Answer from the drawing. Dimensions are ordinates in mm from the lowest x, y and z of the part. A direction names the side the tool comes from. Round coordinates to 2 decimals unless told otherwise and drop trailing zeros. Order: outer loops, then holes, each group sorted by start corner. A loop starts at its lowest first (then second) coordinate and runs counter-clockwise, first axis right, second up. Notation, with made-up numbers: (50, -29) -> (54, -29) arc R15 ccw to (54, 0) -> close; hole circle Ø3 at (-3, 35.5). An arc over 180 degrees is marked (long way). Use a Markdown table: item, result. Add a question column.
1. Section D-D, the plane x = 12 is taken. Give the vertices of the cut face in (y, z), then the cut area to 3 significant figures.
2. The mould has two halves that part along Z. Classify the marked faces 3, 4 and 5: +Z half, -Z half, draft (parallel to the pull), parting line (faces both ways), or undercut.
3. Consider L1, parallel to Z at x = 52, y = 18.5; L2, parallel to X at y = 31, z = 96; L3, parallel to X at y = 28, z = 99. Determine where each line is inside the solid, lowest interval first. Write a range as [from, to].
4. Section C-C, the plane z = 93 is taken. Give the vertices of the cut face in (x, y).
5. For the marked faces 1 and 2, determine the directions among +Z, -Z, +X, -X, +Y, -Y from which every point of the face is accessible in a straight line to the end or side of a thin tool.
6. Given pin 1 (3 mm diameter, centred on x = 7.5, y = 39, fed in from +Z); pin 2 (5 mm diameter, centred on x = 24, z = 34.5, fed in from +Y); pin 3 (10 mm diameter, centred on x = 30.5, z = 37, fed in from +Y), each flat-ended and moving along its own axis, determine where each tip first touches the part or whether it passes through.
7. Section A-A, the plane y = 32 is taken. Give the vertices of the cut face in (x, z), then the cut area to 3 significant figures.
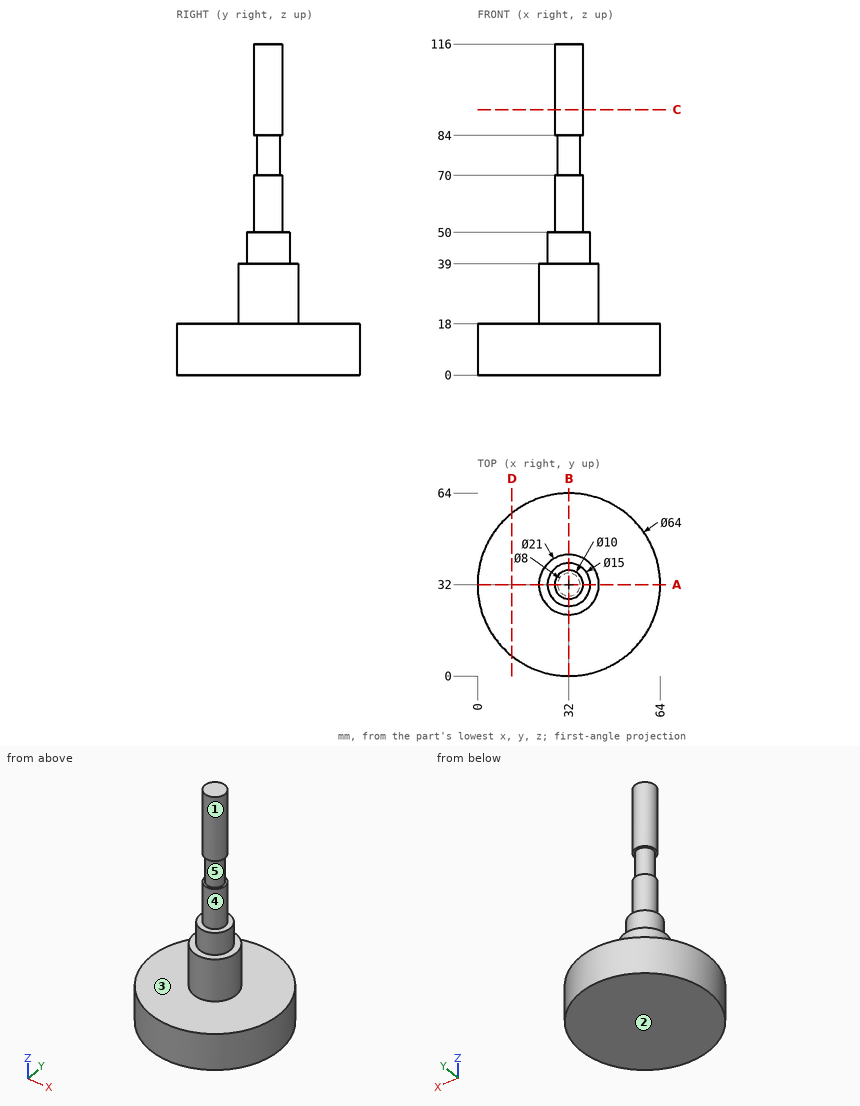
Verdict:
| question | item | result |
|---|---|---|
| 1 | outline | (7.02, 0) -> (56.98, 0) -> (56.98, 18) -> (7.02, 18) -> close |
| 1 | area | 899 mm2 |
| 2 | face 3 | +Z half |
| 2 | face 4 | draft |
| 2 | face 5 | undercut |
| 3 | L1 | z = [0, 18] |
| 3 | L2 | x = [27.1, 36.9] |
| 3 | L3 | x = [29, 35] |
| 4 | outline | circle Ø10 at (32, 32) |
| 5 | face 1 | +Z |
| 5 | face 2 | -Z, +X, -X, +Y, -Y |
| 6 | pin 1 | stops at z = 18 |
| 6 | pin 2 | stops at y = 40.94 |
| 6 | pin 3 | stops at y = 42.5 |
| 7 | outline | (0, 0) -> (64, 0) -> (64, 18) -> (42.5, 18) -> (42.5, 39) -> (39.5, 39) -> (39.5, 50) -> (37, 50) -> (37, 70) -> (36, 70) -> (36, 84) -> (37, 84) -> (37, 116) -> (27, 116) -> (27, 84) -> (28, 84) -> (28, 70) -> (27, 70) -> (27, 50) -> (24.5, 50) -> (24.5, 39) -> (21.5, 39) -> (21.5, 18) -> (0, 18) -> close |
| 7 | area | 2,390 mm2 |
